Geometry check sheet. Reference: the model listing, model coordinates, mm. Give positions to 0.01 mm unless a question says otherwise; leave off trailing zeros. Order: outer loops, then holes, each group sorted by start corner. A loop starts at its lowest first (then second) coordinate and runs counter-clockwise, first axis right, second up. Notation, with made-up numbers: M -8.5,-17.75 L 34.5,-17.75 A16 ccw 34.5,-0.75 Z; hole C 38,84.25 d5. An arc over 180 degrees is marked long. Answer as CSV lines item,"result". Start each with the question number.
```python
from build123d import *

# Parameters (mm, degrees)
SKETCH2_W                    = 82.55
SKETCH2_H                    = 1
F_10_0_1935_DIAMETER_HOLE1_D = 5.999999938
CIRPATTERN3_COUNT            = 4


with BuildPart() as part:
    # Sketch2 → Revolve1 (revolve)
    with BuildSketch(Plane(origin=(0, 0, 0), x_dir=(0, 0, -1), z_dir=(1, 0, 0))):
        with Locations((-41.275, 0.5)):
            Rectangle(SKETCH2_W, SKETCH2_H)
    revolve(axis=Axis((0, -0.05, 0), (0, 1, 0)))

    # #10 (0.1935) Diameter Hole1 (through all)
    with Locations(Plane(origin=(0, 1, 0), x_dir=(1, 0, 0), z_dir=(0, 1, 0))):
        with Locations((-25.333643223, 61.160825052), (264.743675233, 73.787758551), (-67.027460084, 27.763683018), (-25.809397513, 25.809397513)):
            f_10_0_1935_diameter_hole1 = Hole(F_10_0_1935_DIAMETER_HOLE1_D / 2)

    # CirPattern3: #10 (0.1935) Diameter Hole1 ×4 about axis
    cirpattern3_axis = Axis((0, 0, 0), (0, 1, 0))
    for i in range(1, CIRPATTERN3_COUNT):
        add(f_10_0_1935_diameter_hole1.rotate(cirpattern3_axis, i * 360 / CIRPATTERN3_COUNT), mode=Mode.SUBTRACT)


solid = part.part
```
Item 1: Draft check along Z on faces 1 (the face through (-69.89, 0.49, -28.66)), 2 (the face through (-80.587, 0.507, -17.895)), 3 (the face through (22.95, 0.49, 59.34)), 4 (the face through (1, 1, -1)). Enter one of: pulls with the +Z half, pulls with the -Z half, needs draft (parallel to the pull), parting line crosses it, or undercut.
Item 2: Section check C-C on z = 51.5. Record the boundary of the cut face in (x, y).
Item 3: Scan lines: line 1 along Z through (x, y) = (-24, 0.05); line 2 along Z through (x, y) = (-30, 0.45); line 3 along Z through (x, y) = (-69, 0.15). Record each from-to range of solid material in increasing order.
Item 4: Depth check by flat-ended pin: pin 1 Ø3.5 at (x, z) = (-27.76, 67.03) entering from +Y; pin 2 Ø8 at (x, z) = (67.03, 27.76) entering from +Y. Enter the tip coordinate at first touch or a pass-through.
Item 5: Section check A-A on y = 0.15. Give the number of separate pieces and of enclosed holes in the cut face, then the cut area to 3 significant figures.
Item 6: Section check B-B on x = -67.5. Record the boundary of the cut face in (y, z), then the cut area to 3 significant figures.
Numbers:
1,face 1,"undercut"
1,face 2,"parting line crosses it"
1,face 3,"undercut"
1,face 4,"needs draft"
2,outline,"M -64.52,0 L 64.52,0 L 64.52,1 L -64.52,1 Z"
3,line 1,"-78.98 to -63.85, -58.47 to -28.2, -23.42 to 23.42, 28.2 to 78.98"
3,line 2,"-76.91 to 65.03, 69.03 to 76.91"
3,line 3,"-45.32 to -30.02, -25.5 to 45.32"
4,pin 1,"through"
4,pin 2,"y = 1"
5,separate pieces,"1"
5,enclosed holes,"12"
5,area,"21,100 mm2"
6,outline,"M 0,-47.52 L 1,-47.52 L 1,-30.73 L 0,-30.73 Z; M 0,-24.8 L 1,-24.8 L 1,47.52 L 0,47.52 Z"
6,area,"89.1 mm2"
